from build123d import *

# Parameters (mm, degrees)
BOSS_EXTRUDE1_DEPTH = 2.1
SKETCH2_R           = 4.05
BOSS_EXTRUDE2_DEPTH = 7
FILLET1_R           = 0.5
CHAMFER1_SIZE       = 1


with BuildPart() as part:
    # Sketch1 → Boss-Extrude1 (new body)
    with BuildSketch(Plane.XY):
        Polygon((5.281312122, 3.049166975), (0, 6.09833395), (-5.281312122, 3.049166975), (-5.281312122, -3.049166975), (0, -6.09833395), (5.281312122, -3.049166975), align=None)
    extrude(amount=BOSS_EXTRUDE1_DEPTH)

    # Sketch2 → Boss-Extrude2 (add)
    with BuildSketch(Plane.XY.offset(2.1)):
        Circle(SKETCH2_R)
    extrude(amount=BOSS_EXTRUDE2_DEPTH)

    # Fillet1
    fillet1_edges = [part.edges().sort_by_distance(p)[0] for p in [
        (5.281312122, -3.049166975, 1.05),
        (0, -6.09833395, 1.05),
        (-5.281312122, -3.049166975, 1.05),
        (-5.281312122, 3.049166975, 1.05),
        (0, 6.09833395, 1.05),
        (5.281312122, 3.049166975, 1.05),
        (-4.05, 0, 2.1),
    ]]
    fillet(fillet1_edges, radius=FILLET1_R)

    # Chamfer1
    chamfer1_edges = [part.edges().sort_by_distance(p)[0] for p in [
        (-4.05, 0, 9.1),
    ]]
    chamfer(chamfer1_edges, length=CHAMFER1_SIZE)


solid = part.part
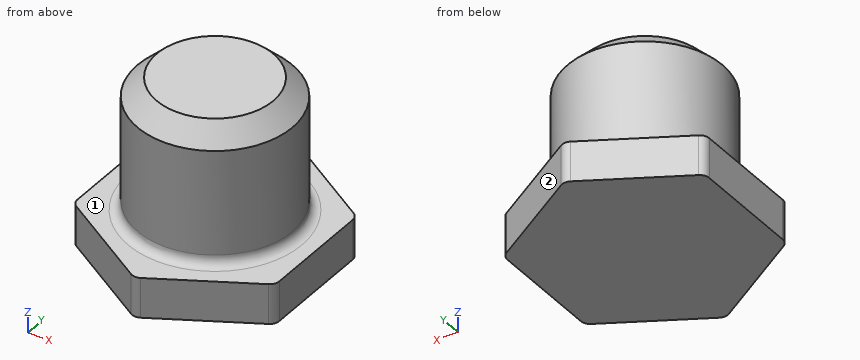
Source: CAD feature listing. Evaluate the final solid. Frame: model axes, mm. Face numbers are marked on the shaded views. A direction names the side the tool comes from. Round coordinates to 2 decimals unless told otherwise and drop trailing zeros. Loops run counter-clockwise (first coordinate to the right, second up) from the corner with the lowest first, then second, coordinate; pieces in that order, holes last. Notation, with made-up numbers: (49, 60) -> (89, 60) arc R14 cw to (89, 67) -> close; hole circle Ø3 at (-36.75, 71). An arc over 180 degrees is marked (long way). Answer as a JSON object with one key per item and string values. Group by question number.
Q1. Section query C-C (z = 3.5). Output: boundary loops of the cut face in (x, y).
Q2. Contact query for flat-ended pins moving along their axis: P1, Ø2, axis at y = -2.5, z = 6, coming from the -X side; P2, Ø2, axis at x = 3.5, z = 3, coming from the -Y side; P3, Ø2, axis at x = -2, z = 3, coming from the -Y side. Output: stop coordinate, or through.
Q3. Access query for the marked faces 1 and 2. Directions: +Z, -Z, +X, -X, +Y, -Y. A direction counts if a zero-diameter tool reaches every point of the face in a straight line with its end or side. Return the directions, or none.
Q4. Section query A-A (z = 1.25). Output: boundary loops of the cut face in (x, y), plus the area to 3 significant figures.
Q5. Section query B-B (x = 0). Output: boundary loops of the cut face in (y, z), plus the area to 3 significant figures.
Q6. Ray query, line 1 (Z direction, x = -2.25, y = 4); line 2 (X direction, y = -2, z = 7.75); line 3 (X direction, y = 1.75, z = 3.5). Return the intervals inside material, ascending. Write a range as from..to.
Completed:
{
 "1": {"outline": "circle Ø8.1 at (0, 0)"},
 "2": {"P1": "x = -3.76", "P2": "y = -4.33", "P3": "y = -5.2"},
 "3": {"face 1": "+Z", "face 2": "+Z, -Z, +X, +Y"},
 "4": {"outline": "(-5.28, -2.76) arc R0.5 ccw to (-5.03, -3.19) -> (-0.25, -5.95) arc R0.5 ccw to (0.25, -5.95) -> (5.03, -3.19) arc R0.5 ccw to (5.28, -2.76) -> (5.28, 2.76) arc R0.5 ccw to (5.03, 3.19) -> (0.25, 5.95) arc R0.5 ccw to (-0.25, 5.95) -> (-5.03, 3.19) arc R0.5 ccw to (-5.28, 2.76) -> close", "area": "96.5 mm²"},
 "5": {"outline": "(-6.02, 0) -> (6.02, 0) -> (6.02, 2.1) -> (4.55, 2.1) arc R0.5 cw to (4.05, 2.6) -> (4.05, 8.1) -> (3.05, 9.1) -> (-3.05, 9.1) -> (-4.05, 8.1) -> (-4.05, 2.6) arc R0.5 cw to (-4.55, 2.1) -> (-6.02, 2.1) -> close", "area": "81.1 mm²"},
 "6": {"line 1": "0..2.1", "line 2": "-3.52..3.52", "line 3": "-3.65..3.65"}
}
